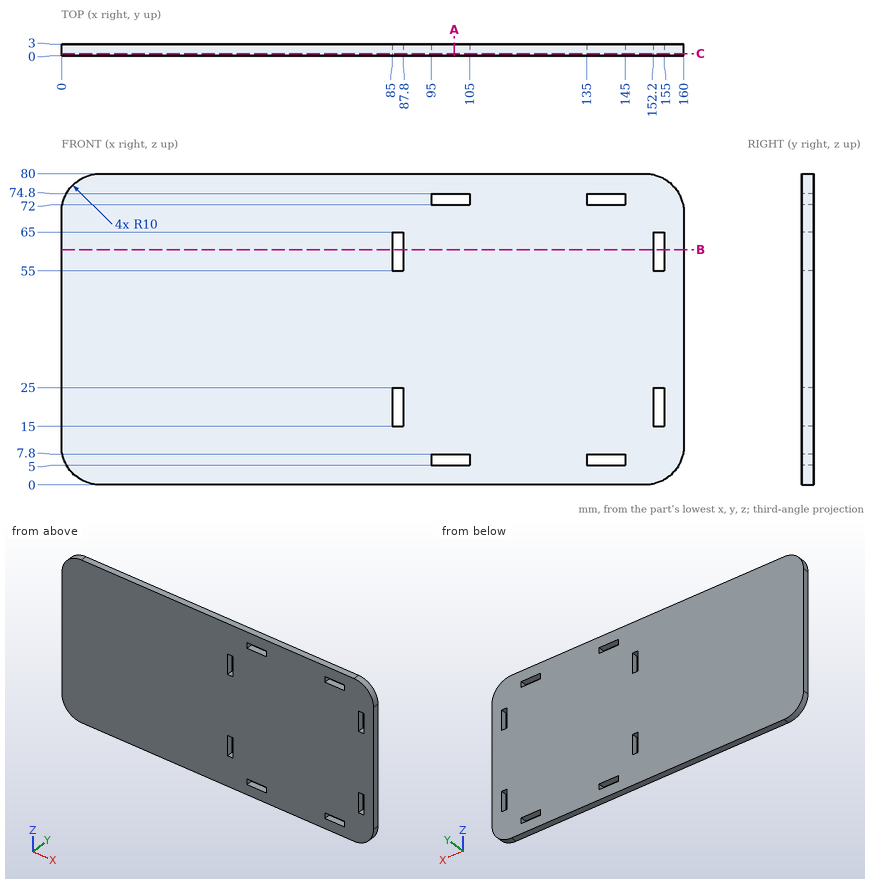
Here's the drawing with two shaded views (mm, measured from the low corner). I have some questions. Give positions to 0.01 mm unless a question says otherwise; leave off trailing zeros. Loops run counter-clockwise (first coordinate to the right, second up) from the corner with the lowest first, then second, coordinate; pieces in that order, holes last. Notation, with made-up numbers: (19, 10) - (56, 10) arc R35 ccw to (56, 47) - close; hole circle Ø2 at (-40, 60). An arc over 180 degrees is marked (long way). Answer in a Markdown table with one row per item. Add a question column.
Q1. If we section it at B-B (z = 60.5): List the corners of the cut face in (x, y) for me, plus the area to 3 significant figures.
Q2. If we section it at C-C (y = 0.5): State how many separate pieces and enclosed holes the cut face has, plus the area to 3 significant figures.
Q3. If we section it at A-A (x = 101): List the corners of the cut face in (y, z) for me, plus the area to 3 significant figures.
Q4. For pin 1 (0.8 mm diameter, centred on y = 1, z = 73, fed in from +X); pin 2 (0.8 mm diameter, centred on y = 1, z = 73.5, fed in from +X); pin 3 (0.8 mm diameter, centred on y = 1, z = 73, fed in from -X), each with a flat end and sliding along its axis, tell me the tip position at first contact or that it passes through.
Q5. Please list where these lines run through material, in increasing order: L1, parallel to X at y = 1.3, z = 60; L2, parallel to Z at x = 96.5, y = 2.3; L3, parallel to Z at x = 85.5, y = 1.05. Write a range as from..to.
The answers:
| question | item | result |
|---|---|---|
| 1 | outline | (0, 0) - (85, 0) - (85, 3) - (0, 3) - close; (87.8, 0) - (152.2, 0) - (152.2, 3) - (87.8, 3) - close; (155, 0) - (160, 0) - (160, 3) - (155, 3) - close |
| 1 | area | 463 mm^2 |
| 2 | separate pieces | 1 |
| 2 | enclosed holes | 8 |
| 2 | area | 12,500 mm^2 |
| 3 | outline | (0, 0) - (3, 0) - (3, 5) - (0, 5) - close; (0, 7.8) - (3, 7.8) - (3, 72) - (0, 72) - close; (0, 74.8) - (3, 74.8) - (3, 80) - (0, 80) - close |
| 3 | area | 223 mm^2 |
| 4 | pin 1 | stops at x = 159.66 |
| 4 | pin 2 | stops at x = 159.51 |
| 4 | pin 3 | stops at x = 0.34 |
| 5 | L1 | x = 0..85, 87.8..152.2, 155..160 |
| 5 | L2 | z = 0..5, 7.8..72, 74.8..80 |
| 5 | L3 | z = 0..15, 25..55, 65..80 |
